Check sheet for the modelled part. Datum: model origin and axes. Units: mm. Give positions to 0.01 mm unless a question says otherwise; leave off trailing zeros. Write each loop counter-clockwise with the first axis right and the second up, starting at its lowest first coordinate (ties: lowest second). Pieces come first, ordered by that corner, then holes.
from build123d import *

# Parameters (mm, degrees)
SKETCH1_W                = 230
SKETCH1_H                = 425
BOSS_EXTRUDE1_DEPTH      = 3
F_5_0_4_DIAMETER_HOLE1_D = 5
SKETCH5_W                = 41.25
SKETCH5_H                = 238.6
CUT_EXTRUDE1_DEPTH       = 4
SKETCH6_W                = 250
SKETCH6_H                = 580
SKETCH6_W_2              = 230
SKETCH6_H_2              = 425
BOSS_EXTRUDE3_DEPTH      = 3


with BuildPart() as part:
    # Sketch1 → Boss-Extrude1 (new body)
    with BuildSketch(Plane(origin=(0, 0, 0), x_dir=(1, 0, 0), z_dir=(0, 1, 0))):
        Rectangle(SKETCH1_W, SKETCH1_H)
    extrude(amount=-BOSS_EXTRUDE1_DEPTH)

    # Ø5.0 (4) Diameter Hole1 (through all)
    with Locations(Plane(origin=(0, 0, 0), x_dir=(1, 0, 0), z_dir=(0, 1, 0))):
        with Locations((-105, 202.5), (105, 202.5), (105, -202.5), (-105, -202.5)):
            Hole(F_5_0_4_DIAMETER_HOLE1_D / 2)

    # Sketch5 → Cut-Extrude1 (cut, through all)
    with BuildSketch(Plane(origin=(0, 0, 0), x_dir=(1, 0, 0), z_dir=(0, 1, 0))):
        with Locations((-40.125, -0.7)):
            Rectangle(SKETCH5_W, SKETCH5_H)
        with Locations((40.125, -0.7)):
            Rectangle(SKETCH5_W, SKETCH5_H)
    extrude(amount=-CUT_EXTRUDE1_DEPTH, mode=Mode.SUBTRACT)

    # Sketch6 → Boss-Extrude3 (add)
    with BuildSketch(Plane(origin=(0, 0, 0), x_dir=(1, 0, 0), z_dir=(0, 1, 0))):
        Rectangle(SKETCH6_W, SKETCH6_H)
        Rectangle(SKETCH6_W_2, SKETCH6_H_2, mode=Mode.SUBTRACT)
    extrude(amount=-BOSS_EXTRUDE3_DEPTH)


solid = part.part
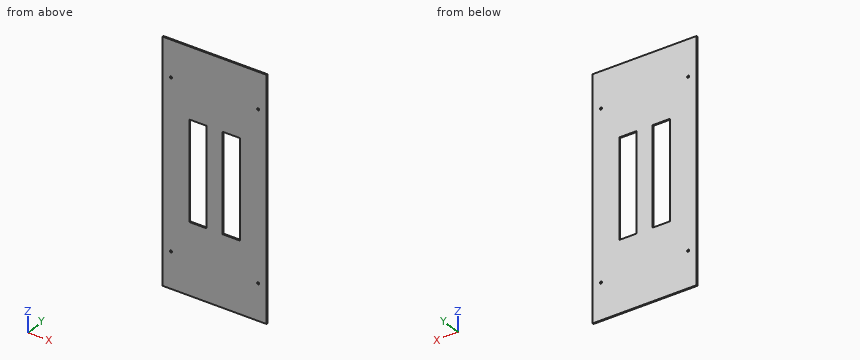
1) Sectioned sample at A-A on x = 42.5. Record the boundary of the cut face in (y, z), then the cut area to 3 significant figures.
2) Scan lines: L1, parallel to Z at x = -105, y = -1.6; L2, parallel to X at y = -1.4, z = 202.5; L3, parallel to X at y = -1, z = -30. Record each from-to range of solid material in increasing order.
3) Sectioned sample at C-C on y = -1.6. Record the boundary of the cut face in (x, z).
4) Gauge pin test, flat end, axial feed: pin 1 (4 mm diameter, centred on x = -105, z = 202.5, fed in from -Y). Record the tip position at first contact, or that the pin passes through.
5) Sectioned sample at B-B on z = 41. Record the boundary of the cut face in (x, y).
Answers below:
1. outline: (-3, -290) - (0, -290) - (0, -118.6) - (-3, -118.6) - close; (-3, 120) - (0, 120) - (0, 290) - (-3, 290) - close
1. area: 1,020 mm2
2. L1: z = -290 to -205, -200 to 200, 205 to 290
2. L2: x = -125 to -107.5, -102.5 to 102.5, 107.5 to 125
2. L3: x = -125 to -60.75, -19.5 to 19.5, 60.75 to 125
3. outline: (-125, -290) - (125, -290) - (125, 290) - (-125, 290) - close; hole circle Ø5 at (-105, -202.5); hole circle Ø5 at (-105, 202.5); hole (-60.75, -118.6) - (-19.5, -118.6) - (-19.5, 120) - (-60.75, 120) - close; hole (19.5, -118.6) - (60.75, -118.6) - (60.75, 120) - (19.5, 120) - close; hole circle Ø5 at (105, -202.5); hole circle Ø5 at (105, 202.5)
4. pin 1: passes through
5. outline: (-125, -3) - (-60.75, -3) - (-60.75, 0) - (-125, 0) - close; (-19.5, -3) - (19.5, -3) - (19.5, 0) - (-19.5, 0) - close; (60.75, -3) - (125, -3) - (125, 0) - (60.75, 0) - close
